Solid Edge part; units mm, degrees
sketch "Sketch1" plane through (0, 0, 0) normal (0, 0, 1) x (1, 0, 0)
  line L0 (40, -25) -> (40, 30)
  line L1 (40, 30) -> (-44, 30)
  line L2 (-44, 30) -> (-44, -25)
  line L3 (-44, -25) -> (40, -25)
extrude "ExtrudedProtrusion_3" add sketch "Sketch1" along normal blind 2
sketch "Sketch2" plane through (0, 0, 0) normal (0, 0, 1) x (1, 0, 0)
  line L0 (-44, 28) -> (-27, 28)
  line L1 (-27, 28) -> (-27, 30)
  line L2 (-27, 30) -> (-44, 30)
  line L3 (-44, 30) -> (-44, 28)
extrude "ExtrudedCutout_9" cut sketch "Sketch2" along normal blind 2
sketch "Sketch3" plane through (0, 0, 0) normal (0, 0, 1) x (1, 0, 0)
  line L0 (-17, 28) -> (13, 28)
  line L1 (13, 28) -> (13, 30)
  line L2 (13, 30) -> (-17, 30)
  line L3 (-17, 30) -> (-17, 28)
extrude "ExtrudedCutout_10" cut sketch "Sketch3" along normal blind 2
sketch "Sketch4" plane through (0, 0, 0) normal (0, 0, 1) x (1, 0, 0)
  line L0 (23, 28) -> (40, 28)
  line L1 (40, 28) -> (40, 30)
  line L2 (40, 30) -> (23, 30)
  line L3 (23, 30) -> (23, 28)
extrude "ExtrudedCutout_11" cut sketch "Sketch4" along normal blind 2
sketch "Sketch5" plane through (0, 0, 0) normal (0, 0, 1) x (1, 0, 0)
  line L0 (38, -2.5) -> (38, 7.5)
  line L1 (38, 7.5) -> (36, 7.5)
  line L2 (36, 7.5) -> (36, -2.5)
  line L3 (36, -2.5) -> (38, -2.5)
extrude "ExtrudedCutout_12" cut sketch "Sketch5" along normal blind 2
sketch "Sketch6" plane through (0, 0, 0) normal (0, 0, 1) x (1, 0, 0)
  line L0 (40, -23) -> (23, -23)
  line L1 (23, -23) -> (23, -25)
  line L2 (23, -25) -> (40, -25)
  line L3 (40, -25) -> (40, -23)
extrude "ExtrudedCutout_13" cut sketch "Sketch6" along normal blind 2
sketch "Sketch7" plane through (0, 0, 0) normal (0, 0, 1) x (1, 0, 0)
  line L0 (13, -23) -> (-17, -23)
  line L1 (-17, -23) -> (-17, -25)
  line L2 (-17, -25) -> (13, -25)
  line L3 (13, -25) -> (13, -23)
extrude "ExtrudedCutout_14" cut sketch "Sketch7" along normal blind 2
sketch "Sketch8" plane through (0, 0, 0) normal (0, 0, 1) x (1, 0, 0)
  line L0 (-27, -23) -> (-44, -23)
  line L1 (-44, -23) -> (-44, -25)
  line L2 (-44, -25) -> (-27, -25)
  line L3 (-27, -25) -> (-27, -23)
extrude "ExtrudedCutout_15" cut sketch "Sketch8" along normal blind 2
sketch "Sketch9" plane through (0, 0, 0) normal (0, 0, 1) x (1, 0, 0)
  line L0 (-40, -2.5) -> (-40, 7.5)
  line L1 (-40, 7.5) -> (-42, 7.5)
  line L2 (-42, 7.5) -> (-42, -2.5)
  line L3 (-42, -2.5) -> (-40, -2.5)
extrude "ExtrudedCutout_16" cut sketch "Sketch9" along normal blind 2
fillet "Round_1" radius 1 1 edges at (-44, -23, 1)
fillet "Round_2" radius 1 3 edges at (-44, 28, 1) (40, 28, 1) (40, -23, 1)
properties material "Acrylic, high impact grade"
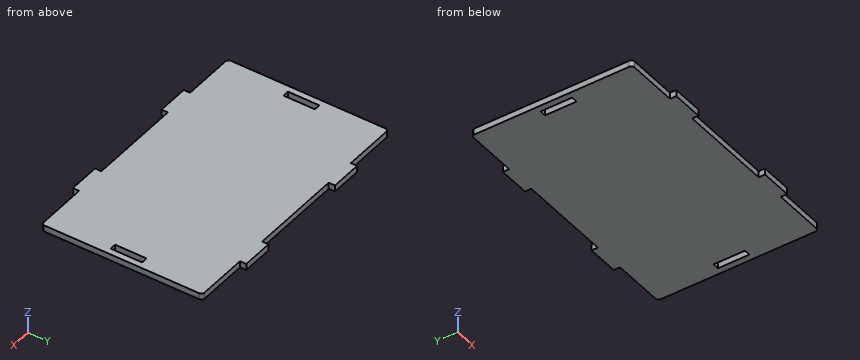
Model file for the job. Use its own axes, mm. Coordinates: 2 decimals unless noted, no trailing zeros. Loops run counter-clockwise (first coordinate to the right, second up) from the corner with the lowest first, then second, coordinate; pieces in that order, holes last. Notation, with made-up numbers: (32.5, 89) -> (49.5, 89) arc R19 cw to (49.5, 112) -> close; hole circle Ø2 at (9.5, 44.5). An arc over 180 degrees is marked (long way). Use one line per item in the form item = value. Start each with the question number.
(1) Probe probe 1 along X at (y, z) = (5, 0.7); probe 2 along Y at (x, z) = (-16.5, 0.75). List the from-to ranges inside material, lowest first. Write a range as from..to.
(2) Cut at A-A on y = 6.5. Give the cut face in (x, z).
(3) Flat gauge pins, fed straight in: pin 1 (1 mm diameter, centred on y = 29, z = 0.5, fed in from -X); pin 2 (12 mm diameter, centred on x = 14.5, y = -11, fed in from -Z); pin 3 (1 mm diameter, centred on x = -6.5, z = 0.5, fed in from +Y); pin 4 (0.6 mm diameter, centred on x = -1, z = 1.5, fed in from -Y). Where does each tip first touch, or does it go through?
(4) Cut at C-C on x = 34. Give the cut face in (y, z), and give its area (3 significant figures).
(5) Cut at B-B on z = 0.95. Give the number of separate pieces and of enclosed holes in the cut face, and give its area (3 significant figures).
Values:
q1.probe_1 = -44..-42, -40..36, 38..40
q1.probe_2 = -23..28
q2.outline = (-44, 0) -> (-42, 0) -> (-42, 2) -> (-44, 2) -> close; (-40, 0) -> (36, 0) -> (36, 2) -> (-40, 2) -> close; (38, 0) -> (40, 0) -> (40, 2) -> (38, 2) -> close
q3.pin_1 = -27
q3.pin_2 = 0
q3.pin_3 = 28
q3.pin_4 = -23
q4.outline = (-23, 0) -> (28, 0) -> (28, 2) -> (-23, 2) -> close
q4.area = 102 mm2
q5.separate_pieces = 1
q5.enclosed_holes = 2
q5.area = 4,320 mm2
